```python
from build123d import *

# Parameters (mm, degrees)
F1_DEPTH = 25.4


with BuildPart() as f1:
    # F0 (on Right) → F1 (new body)
    with BuildSketch(Plane.YZ):
        Polygon((-23.609508, 44.494845), (-23.609508, -44.494845), (23.609508, -44.494845), (23.609508, 44.494845), (2.825069, 55.795118), (2.825069, 64.472117), (0, 64.472117), (-2.825069, 64.472117), (-2.825069, 55.795118), align=None)
    extrude(amount=F1_DEPTH)


solid = f1.part
```
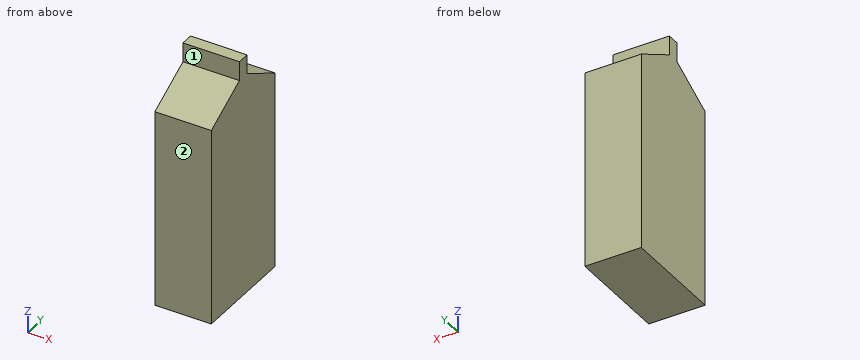
Read the model definition and answer for the solid it produces. Units are mm, in the model's axes. Face numbers are marked on the shaded views. A direction names the side the tool comes from. Round coordinates to 2 decimals unless told otherwise and drop trailing zeros. Write each loop counter-clockwise with the first axis right and the second up, starting at its lowest first coordinate (ties: lowest second). Pieces come first, ordered by that corner, then holes. Notation, with made-up numbers: M 56,38 L 74,38 A13 cw 74,60 Z; hole C 63,-21 d9. An arc over 180 degrees is marked long. One line per item, written item: value.
Q1. Find section A-A on x = 8.25. Write down the section's boundary in (y, z), plus the area to 3 significant figures.
Data:
outline: M -23.61,-44.49 L 23.61,-44.49 L 23.61,44.49 L 2.83,55.8 L 2.83,64.47 L -2.83,64.47 L -2.83,55.8 L -23.61,44.49 Z
area: 4,550 mm2
Q2. Find section B-B on y = 20. Write down the section's boundary in (x, z).
Data:
outline: M 0,-44.49 L 25.4,-44.49 L 25.4,46.46 L 0,46.46 Z
Q3. Which of the six approach directions +Z, -Z, +X, -X, +Y, -Y give full straight-line access (tool end or side, diameter ignored) to the marked faces 1 and 2?
Data:
face 1: +Z, +X, -X, -Y
face 2: +Z, -Z, +X, -X, -Y
Q4. Find section C-C on y = -13. Write down the section's boundary in (x, z).
Data:
outline: M 0,-44.49 L 25.4,-44.49 L 25.4,50.26 L 0,50.26 Z
Q5. Flat-ended cylindrical pins translate along their axes: pin 1 Ø7 at (x, z) = (7, 60) entering from +Y; pin 2 Ø7 at (x, z) = (18, 58.5) entering from -Y. Find the tip coordinate at first contact, or state that the pin passes through.
Data:
pin 1: y = 2.83
pin 2: y = -4.29
Q6. Straight lines are drawn through the part: line 1 (Y direction, x = 19, z = 50); line 2 (Z direction, x = 6.25, y = -10.5); line 3 (Z direction, x = 18, y = 6.5). For each, find the intervals that lie inside material, in ascending order. Write a range as [from, to].
Data:
line 1: [-13.48, 13.48]
line 2: [-44.49, 51.62]
line 3: [-44.49, 53.8]
